```python
from build123d import *

# Parameters (mm, degrees)
F0_R     = 6.35
F0_R_2   = 5.207
F1_DEPTH = 6.35
F2_R     = 7.7175141939
F2_R_2   = 6.35
F3_DEPTH = 2.54
F4_DEPTH = 2.54


with BuildPart() as f1:
    # F0 (on Top) → F1 (new body)
    with BuildSketch(Plane.XY):
        Circle(F0_R)
        Circle(F0_R_2, mode=Mode.SUBTRACT)
    extrude(amount=F1_DEPTH)

    # F2 (on face) → F3 (join)
    with BuildSketch(Plane.XY.offset(6.35)):
        Circle(F2_R)
        Circle(F2_R_2, mode=Mode.SUBTRACT)
    extrude(amount=F3_DEPTH)

    # F4 (add): a face of the model
    f4_faces = [f1.faces().sort_by_distance(p)[0] for p in [
        (-6.1703948776, 0, 6.35),
    ]]
    extrude(f4_faces, amount=F4_DEPTH)


solid = f1.part
```
Check sheet for the modelled part. Datum: model origin and axes. Units: mm. A direction names the side the tool comes from. Round coordinates to 2 decimals unless told otherwise and drop trailing zeros. Loops run counter-clockwise (first coordinate to the right, second up) from the corner with the lowest first, then second, coordinate; pieces in that order, holes last. Notation, with made-up numbers: (48.25, -20) -> (88.25, -20) arc R18 cw to (88.25, 0) -> close; hole circle Ø6 at (57.25, 87.5). An arc over 180 degrees is marked (long way). Write item = value, one per line. Start each with the question number.
1) Set-up check for faces 4 (the cylindrical face through (-1.38, -6.2, 3.13)), 5 (the flat face through (-5, 2, 0)): record each of +Z, -Z, +X, -X, +Y, -Y from which the full face is reachable in a straight line by a thin tool's end or side.
2) Sectioned sample at A-A, the plane x = 0. Record the cut outline in (y, z), plus the area to 3 significant figures.
3) Gauge pin test, flat ends, axial feed: pin 1 Ø4 at (y, z) = (3.5, 7.5) entering from +X; pin 2 Ø1.5 at (y, z) = (0, 3.5) entering from +X; pin 3 Ø3 at (x, z) = (-2, 4) entering from -Y. Record the tip position at first contact, or that the pin passes through.
4) Release check for a two-part mould opening along Y. For faces 1 (the cylindrical face through (-1.005, 7.652, 7.602)), 2 (the flat face through (2, -5, 8.89)), 3 (the cylindrical face through (4.967, 1.564, 4.383)) record: released by +Y, released by -Y, zero draft, split by the parting line, or undercut.
5) Sectioned sample at C-C, the plane y = 6. Record the cut outline in (x, z), plus the area to 3 significant figures.
6) Sectioned sample at D-D, the plane z = 2. Record the cut outline in (x, y).
7) Thickness scan on probe 1 along Y at (x, z) = (0, 5.5); probe 2 along Y at (x, z) = (0, 7); probe 3 along X at (y, z) = (-1.25, 7.75). Record the ranges inside material, lowest first.
Results are:
q1.face_4 = -Z
q1.face_5 = -Z, +X, -X, +Y, -Y
q2.outline = (-7.72, 6.35) -> (-6.35, 6.35) -> (-6.35, 0) -> (-5.21, 0) -> (-5.21, 8.89) -> (-7.72, 8.89) -> close; (5.21, 0) -> (6.35, 0) -> (6.35, 6.35) -> (7.72, 6.35) -> (7.72, 8.89) -> (5.21, 8.89) -> close
q2.area = 27.3 mm^2
q3.pin_1 = 7.57
q3.pin_2 = 6.35
q3.pin_3 = -6.33
q4.face_1 = split by the parting line
q4.face_2 = zero draft
q4.face_3 = undercut
q5.outline = (-4.85, 6.35) -> (-2.08, 6.35) -> (-2.08, 0) -> (2.08, 0) -> (2.08, 6.35) -> (4.85, 6.35) -> (4.85, 8.89) -> (-4.85, 8.89) -> close
q5.area = 51.1 mm^2
q6.outline = circle Ø12.7 at (0, 0); hole circle Ø10.41 at (0, 0)
q7.probe_1 = -6.35 to -5.21, 5.21 to 6.35
q7.probe_2 = -7.72 to -5.21, 5.21 to 7.72
q7.probe_3 = -7.62 to -5.05, 5.05 to 7.62
